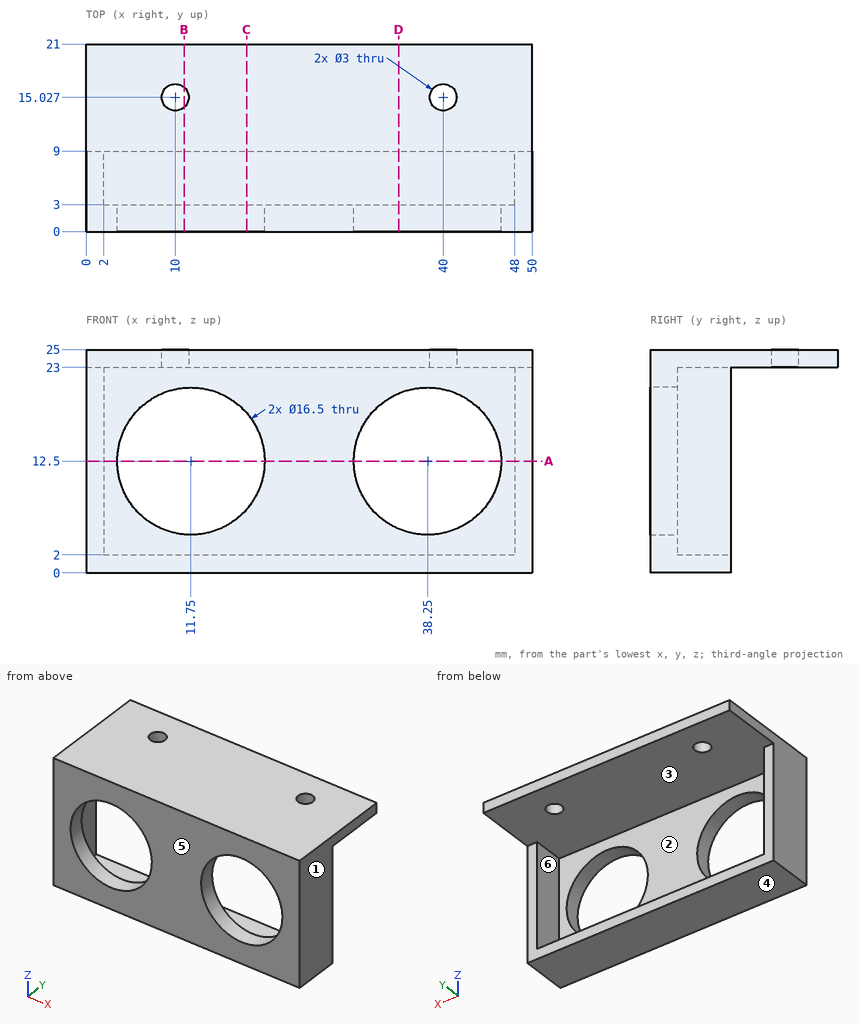
Could you check a few things on this drawing? It's one solid part, dimensions in mm from its lowest x, y, z. A direction names the side the tool comes from. Coordinates: 2 decimals unless noted, no trailing zeros. Order: outer loops, then holes, each group sorted by start corner. A loop starts at its lowest first (then second) coordinate and runs counter-clockwise, first axis right, second up.
1. If we section it at B-B (x = 11): Please give me the cut outline in (y, z) (1 decimal).
2. I'm going to push flat-ended pins straight in: pin 1 (2 mm diameter, centred on x = 18, z = 13.5, fed in from -Y) (1 decimal); pin 2 (6.5 mm diameter, centred on x = 23, z = 11, fed in from +Y); pin 3 (12 mm diameter, centred on x = 39.5, y = 15.5, fed in from -Z). Where does each tip first touch, or does it pass through?
3. If we section it at D-D (x = 35): Please give me the cut outline in (y, z).
4. For the marked faces 1 and 2, which set-ups out of +Z, -Z, +X, -X, +Y, -Y let a thin tool reach every point of the face, with its end or its side?
5. If we section it at A-A (z = 12.5): Please give me the cut outline in (x, y).
6. I need wall thicknesses on line 1 (X direction, y = 2.45, z = 12.5); line 2 (Y direction, x = 10, z = 23.4); line 3 (Z direction, x = 17, y = 5). Which ranges of each line are inside material? Lowest first, please.
7. Thinking about a two-plate mould opening in Z: for the marked faces 3, 4, 5 and 6, which applies, +Z half, -Z half, draft (parallel to the pull), parting line (faces both ways), or undercut?
8. If we section it at C-C (x = 18): Please give me the cut outline in (y, z) (1 decimal).
Entries:
1. outline: (0, 0) - (9, 0) - (9, 2) - (3, 2) - (3, 4.3) - (0, 4.3) - close; (0, 20.7) - (3, 20.7) - (3, 23) - (13.9, 23) - (13.9, 25) - (0, 25) - close; (16.1, 23) - (21, 23) - (21, 25) - (16.1, 25) - close
2. pin 1: passes through
2. pin 2: stops at y = 3
2. pin 3: stops at z = 23
3. outline: (0, 0) - (9, 0) - (9, 2) - (3, 2) - (3, 4.92) - (0, 4.92) - close; (0, 20.08) - (3, 20.08) - (3, 23) - (21, 23) - (21, 25) - (0, 25) - close
4. face 1: +Z, -Z, +X, +Y, -Y
4. face 2: +Y
5. outline: (0, 0) - (3.5, 0) - (3.5, 3) - (2, 3) - (2, 9) - (0, 9) - close; (20, 0) - (30, 0) - (30, 3) - (20, 3) - close; (46.5, 0) - (50, 0) - (50, 9) - (48, 9) - (48, 3) - (46.5, 3) - close
6. line 1: x = 0 to 3.5, 20 to 30, 46.5 to 50
6. line 2: y = 0 to 13.53, 16.53 to 21
6. line 3: z = 0 to 2, 23 to 25
7. face 3: undercut
7. face 4: -Z half
7. face 5: draft
7. face 6: undercut
8. outline: (0, 0) - (9, 0) - (9, 2) - (3, 2) - (3, 7.1) - (0, 7.1) - close; (0, 17.9) - (3, 17.9) - (3, 23) - (21, 23) - (21, 25) - (0, 25) - close
